Source: CAD feature listing. Evaluate the final solid. Frame: model axes, mm. A direction names the side the tool comes from. Give positions to 0.01 mm unless a question says otherwise; leave off trailing zeros. Loops run counter-clockwise (first coordinate to the right, second up) from the corner with the lowest first, then second, coordinate; pieces in that order, holes last. Notation, with made-up numbers: (30, 15.25) -> (87, 15.25) arc R15 cw to (87, 33.25) -> close; hole circle Ø7 at (36, 0.25). An arc over 180 degrees is marked (long way). Return JSON: item names as keys, results as strings. Group by question number.
(1) Cut plane D-D on y = 0. Return loops of the section in (x, z), then the cut area to 3 significant figures.
(2) Pin query (flat end, axial travel): pin 1 (6.5 mm diameter, centred on x = 0, y = 0, fed in from -Z); pin 2 (2.5 mm diameter, centred on y = 3.175, z = 12.7, fed in from +X); pin 3 (1.2 mm diameter, centred on y = 4, z = -12, fed in from -X); pin 4 (2.5 mm diameter, centred on x = 0, y = 0, fed in from +Z). Return the tip coordinate at first contact, or that it passes through.
(3) Cut plane B-B on x = 6. Return loops of the section in (y, z) (3 decimals), then the cut area to 3 significant figures.
(4) Ray query, line 1 (X direction, y = 5.5, z = 0); line 2 (Y direction, x = 0, z = 17.25) (3 decimals); line 3 (X direction, y = 3.75, z = -11). Return the intervals inside material, ascending. Write a range as from..to.
(5) Draft query along X for faces 1 (the face through (-1.926, 0.607, -19.047)), 2 (the face through (-4.166, 3, 13)), 3 (the face through (1.926, 6.394, -0.607)), 4 (the face through (0, -9.525, 0)). Return one class per face: released by +X, released by -X, zero draft, split by the parting line, or undercut.
(6) Cut plane A-A on y = 7. Return loops of the section in (x, z).
(7) Access query for faces 5 (the face through (0, 3.175, 0)), 6 (the face through (10.516, 0, 0)), 7 (the face through (-7.385, 1.946, 11.098)), 8 (the face through (4.166, 3, -13)), 9 (the face through (-0.1, 2.3, 23.743)). Directions: +Z, -Z, +X, -X, +Y, -Y. A direction counts if a zero-diameter tool reaches every point of the face in a straight line with its end or side. Return the directions, or none.
(8) Cut plane C-C on z = -12.7. Return loops of the section in (x, y) (3 decimals), then the cut area to 3 significant figures.
```python
from build123d import *

# Parameters (mm, degrees)
SKETCH1_W           = 21.0312
SKETCH1_H           = 47.4853
BOSS_EXTRUDE1_DEPTH = 9.525
SKETCH2_R           = 2.0193
CUT_EXTRUDE1_DEPTH  = 9.525
SKETCH3_R           = 2.0193
CUT_EXTRUDE2_DEPTH  = 9.525
SKETCH4_R           = 2.0193
CUT_EXTRUDE3_DEPTH  = 6.35
SKETCH5_R           = 2.0193
CUT_EXTRUDE4_DEPTH  = 6.35
SKETCH6_R           = 2.0193
CUT_EXTRUDE5_DEPTH  = 6.35
FILLET1_R           = 2.54


with BuildPart() as part:
    # Sketch1 → Boss-Extrude1 (new body, symmetric)
    with BuildSketch(Plane(origin=(0, 0, 0), x_dir=(1, 0, 0), z_dir=(0, 1, 0))):
        Rectangle(SKETCH1_W, SKETCH1_H)
    extrude(amount=BOSS_EXTRUDE1_DEPTH, both=True)

    # Sketch2 → Cut-Extrude1 (cut)
    with BuildSketch(Plane.XY.offset(23.74265)):
        Circle(SKETCH2_R)
    extrude(amount=-CUT_EXTRUDE1_DEPTH, mode=Mode.SUBTRACT)

    # Sketch3 → Cut-Extrude2 (cut)
    with BuildSketch(Plane(origin=(0, 0, -23.74265), x_dir=(-1, 0, 0), z_dir=(0, 0, -1))):
        Circle(SKETCH3_R)
    extrude(amount=-CUT_EXTRUDE2_DEPTH, mode=Mode.SUBTRACT)

    # Sketch4 → Cut-Extrude3 (cut)
    with BuildSketch(Plane(origin=(10.5156, 0, 0), x_dir=(0, 0, -1), z_dir=(1, 0, 0))):
        with Locations((-12.7, 3.175)):
            Circle(SKETCH4_R)
        with Locations((12.7, 3.175)):
            Circle(SKETCH4_R)
        with Locations((0, 3.175)):
            Circle(SKETCH4_R)
    extrude(amount=-CUT_EXTRUDE3_DEPTH, mode=Mode.SUBTRACT)

    # Sketch5 → Cut-Extrude4 (cut)
    with BuildSketch(Plane.ZY.offset(10.5156)):
        with Locations((-12.7, 3.175)):
            Circle(SKETCH5_R)
        with Locations((0, 3.175)):
            Circle(SKETCH5_R)
        with Locations((12.7, 3.175)):
            Circle(SKETCH5_R)
    extrude(amount=-CUT_EXTRUDE4_DEPTH, mode=Mode.SUBTRACT)

    # Sketch6 → Cut-Extrude5 (cut)
    with BuildSketch(Plane(origin=(0, 9.525, 0), x_dir=(1, 0, 0), z_dir=(0, 1, 0))):
        with Locations((0, 12.7)):
            Circle(SKETCH6_R)
        Circle(SKETCH6_R)
        with Locations((0, -12.7)):
            Circle(SKETCH6_R)
    extrude(amount=-CUT_EXTRUDE5_DEPTH, mode=Mode.SUBTRACT)

    # Fillet1
    fillet1_edges = [part.edges().sort_by_distance(p)[0] for p in [
        (10.5156, 0, 23.74265),
        (-10.5156, 0, 23.74265),
        (-10.5156, 0, -23.74265),
        (10.5156, 0, -23.74265),
    ]]
    fillet(fillet1_edges, radius=FILLET1_R)


solid = part.part
```
Answers:
{
 "1": {"outline": "(-10.52, -21.2) arc R2.54 ccw to (-7.98, -23.74) -> (-2.02, -23.74) -> (-2.02, -14.22) -> (2.02, -14.22) -> (2.02, -23.74) -> (7.98, -23.74) arc R2.54 ccw to (10.52, -21.2) -> (10.52, 21.2) arc R2.54 ccw to (7.98, 23.74) -> (2.02, 23.74) -> (2.02, 14.22) -> (-2.02, 14.22) -> (-2.02, 23.74) -> (-7.98, 23.74) arc R2.54 ccw to (-10.52, 21.2) -> close", "area": "916 mm²"},
 "2": {"pin 1": "z = -23.74", "pin 2": "x = 4.17", "pin 3": "x = -4.17", "pin 4": "z = 14.22"},
 "3": {"outline": "(-9.525, -23.743) -> (9.525, -23.743) -> (9.525, 23.743) -> (-9.525, 23.743) -> close; hole circle Ø4.039 at (3.175, -12.7); hole circle Ø4.039 at (3.175, 0); hole circle Ø4.039 at (3.175, 12.7)", "area": "866 mm²"},
 "4": {"line 1": "-10.52..-2.02, 2.02..10.52", "line 2": "-9.525..-2.019, 2.019..9.525", "line 3": "-4.17..-1.09, 1.09..4.17"},
 "5": {"face 1": "undercut", "face 2": "released by -X", "face 3": "undercut", "face 4": "zero draft"},
 "6": {"outline": "(-10.52, -21.2) arc R2.54 ccw to (-7.98, -23.74) -> (7.98, -23.74) arc R2.54 ccw to (10.52, -21.2) -> (10.52, 21.2) arc R2.54 ccw to (7.98, 23.74) -> (-7.98, 23.74) arc R2.54 ccw to (-10.52, 21.2) -> close; hole circle Ø4.04 at (0, -12.7); hole circle Ø4.04 at (0, 0); hole circle Ø4.04 at (0, 12.7)"},
 "7": {"face 5": "+Y", "face 6": "+Z, -Z, +X, +Y, -Y", "face 7": "-X", "face 8": "+X", "face 9": "+Z, +X, -X, +Y, -Y"},
 "8": {"outline": "(-10.516, -9.525) -> (10.516, -9.525) -> (10.516, 1.156) -> (4.166, 1.156) -> (4.166, 5.194) -> (10.516, 5.194) -> (10.516, 9.525) -> (2.019, 9.525) -> (2.019, 3.175) -> (-2.019, 3.175) -> (-2.019, 9.525) -> (-10.516, 9.525) -> (-10.516, 5.194) -> (-4.166, 5.194) -> (-4.166, 1.156) -> (-10.516, 1.156) -> close", "area": "324 mm²"}
}
